Check sheet for the drawn part. Datum: minimum x, y, z corner. Units: mm. A direction names the side the tool comes from. Give positions to 0.01 mm unless a question says otherwise; leave off trailing zeros. Write each loop counter-clockwise with the first axis right and the second up, starting at its lowest first coordinate (ties: lowest second). Pieces come first, ordered by that corner, then holes. Notation, with made-up numbers: M 10,23 L 59,23 A29 ccw 59,53 Z; hole C -24,74.5 d1. An arc over 180 degrees is marked long. Write item = value, one per line.
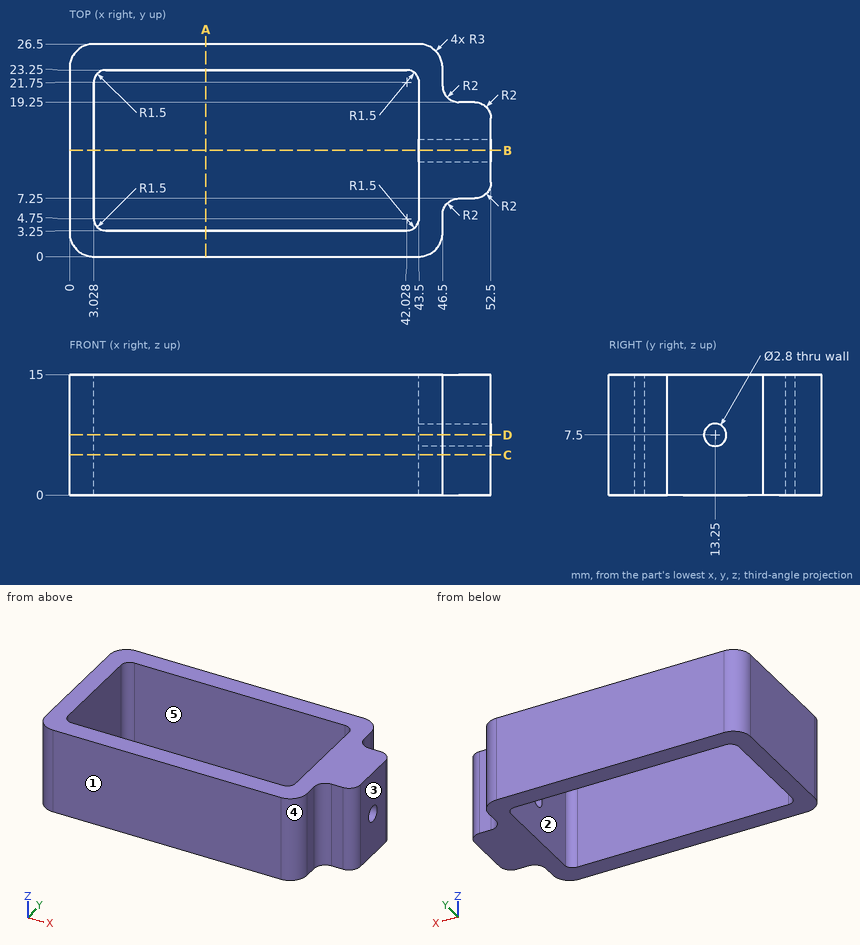
1) Depth check by flat-ended pin: P1, Ø1, axis at y = 7, z = 11, coming from the +X side; P2, Ø3, axis at y = 21.5, z = 5, coming from the +X side; P3, Ø0.7, axis at y = 4, z = 7, coming from the +X side. Enter the tip coordinate at first touch or a pass-through.
From the geometry:
P1 = 51.47
P2 = 46.94
P3 = 46.5
2) Cross-section at C-C on z = 5. Record the boundary of the cut face in (x, y), plus the area to 3 significant figures.
From the geometry:
outline = M 0,3 A3 ccw 3,0 L 43.5,0 A3 ccw 46.5,3 L 46.5,5.25 A2 cw 48.5,7.25 L 50.5,7.25 A2 ccw 52.5,9.25 L 52.5,17.25 A2 ccw 50.5,19.25 L 48.5,19.25 A2 cw 46.5,21.25 L 46.5,23.5 A3 ccw 43.5,26.5 L 3,26.5 A3 ccw 0,23.5 Z; hole M 3.03,4.75 A1.5 ccw 4.53,3.25 L 42.03,3.25 A1.5 ccw 43.5,4.46 L 43.5,22.04 A1.5 ccw 42.03,23.25 L 4.53,23.25 A1.5 ccw 3.03,21.75 Z
area = 489 mm^2
3) Draft check along X on the marked faces 1, 2 and 3. Enter one of: +X half, -X half, draft (parallel to the pull), parting line (faces both ways), or undercut.
From the geometry:
face_1 = draft
face_2 = undercut
face_3 = +X half
4) Cross-section at A-A on x = 17. Record the boundary of the cut face in (y, z), plus the area to 3 significant figures.
From the geometry:
outline = M 0,0 L 3.25,0 L 3.25,15 L 0,15 Z; M 23.25,0 L 26.5,0 L 26.5,15 L 23.25,15 Z
area = 97.5 mm^2
5) Material ranges on probe 1 along X at (y, z) = (21.25, 6.5); probe 2 along Y at (x, z) = (40, 2); probe 3 along Y at (x, z) = (48.75, 7.5), recorded low to high. Write a range as from..to.
From the geometry:
probe_1 = 0..3.03, 43.5..46.5
probe_2 = 0..3.25, 23.25..26.5
probe_3 = 7.25..11.85, 14.65..19.25
6) Cross-section at B-B on y = 13.25. Record the boundary of the cut face in (x, z).
From the geometry:
outline = M 0,0 L 3.03,0 L 3.03,15 L 0,15 Z; M 43.5,0 L 52.5,0 L 52.5,6.1 L 43.5,6.1 Z; M 43.5,8.9 L 52.5,8.9 L 52.5,15 L 43.5,15 Z
7) Tool access check on the marked faces 4 and 5. Record the directions out of +Z, -Z, +X, -X, +Y, -Y that give a thin tool (end or side, any length) a straight path to the whole face; none if there is none.
From the geometry:
face_4 = +Z, -Z, +X, -Y
face_5 = +Z, -Z
8) Cross-section at D-D on z = 7.5. Record the boundary of the cut face in (x, y), plus the area to 3 significant figures.
From the geometry:
outline = M 0,3 A3 ccw 3,0 L 43.5,0 A3 ccw 46.5,3 L 46.5,5.25 A2 cw 48.5,7.25 L 50.5,7.25 A2 ccw 52.5,9.25 L 52.5,11.85 L 43.5,11.85 L 43.5,4.46 A1.5 cw 42.03,3.25 L 4.53,3.25 A1.5 cw 3.03,4.75 L 3.03,21.75 A1.5 cw 4.53,23.25 L 42.03,23.25 A1.5 cw 43.5,22.04 L 43.5,14.65 L 52.5,14.65 L 52.5,17.25 A2 ccw 50.5,19.25 L 48.5,19.25 A2 cw 46.5,21.25 L 46.5,23.5 A3 ccw 43.5,26.5 L 3,26.5 A3 ccw 0,23.5 Z
area = 464 mm^2
